from build123d import *

# Parameters (mm, degrees)
F0_W     = 29
F0_H     = 20
F0_W_2   = 10
F0_H_2   = 5.5
F0_W_3   = 2
F0_W_4   = 57.5
F0_H_3   = 44
F1_DEPTH = 4
F2_DEPTH = 47
F3_R     = 11
F3_R_2   = 1.5
F4_DEPTH = 25
F6_DEPTH = 12.5
F8_DEPTH = 50
F9_R     = 2.5
F10_R    = 5


with BuildPart() as f1:
    # F0 (on Top) → F1 (new body)
    with BuildSketch(Plane.XY):
        with Locations((15.5, -34)):
            Rectangle(F0_W, F0_H)
        with Locations((15, -34)):
            Rectangle(F0_W_2, F0_H_2, mode=Mode.SUBTRACT)
        Polygon((1, -24), (30, -24), (30, 24), (1, 24), (-1, 24), (-30, 24), (-30, 22), (27.5, 22), (27.5, -22), (-30, -22), (-30, -24), (-1, -24), align=None)
        with Locations((0, -34)):
            Rectangle(F0_W_3, F0_H)
        with Locations((15.5, 34)):
            Rectangle(F0_W, F0_H)
        with Locations((15, 34)):
            Rectangle(F0_W_2, F0_H_2, mode=Mode.SUBTRACT)
        with Locations((-15.5, -34)):
            Rectangle(F0_W, F0_H)
        with Locations((-15, -34)):
            Rectangle(F0_W_2, F0_H_2, mode=Mode.SUBTRACT)
        with Locations((0, 34)):
            Rectangle(F0_W_3, F0_H)
        with Locations((-15.5, 34)):
            Rectangle(F0_W, F0_H)
        with Locations((-15, 34)):
            Rectangle(F0_W_2, F0_H_2, mode=Mode.SUBTRACT)
        with Locations((-1.25, 0)):
            Rectangle(F0_W_4, F0_H_3)
    extrude(amount=F1_DEPTH)

    # F0 (on Top) → F2 (join)
    with BuildSketch(Plane.XY):
        Polygon((1, -24), (30, -24), (30, 24), (1, 24), (-1, 24), (-30, 24), (-30, 22), (27.5, 22), (27.5, -22), (-30, -22), (-30, -24), (-1, -24), align=None)
        with Locations((0, 34)):
            Rectangle(F0_W_3, F0_H)
        with Locations((0, -34)):
            Rectangle(F0_W_3, F0_H)
    extrude(amount=F2_DEPTH)

    # F3 (on face) → F4 (cut)
    with BuildSketch(Plane.YZ.offset(30)):
        with Locations((0, 25.5)):
            Circle(F3_R)
        with Locations((-15.5, 41)):
            Circle(F3_R_2)
        with Locations((15.5, 41)):
            Circle(F3_R_2)
        with Locations((15.5, 10)):
            Circle(F3_R_2)
        with Locations((-15.5, 10)):
            Circle(F3_R_2)
    extrude(amount=-F4_DEPTH, mode=Mode.SUBTRACT)

    # F5 (on Right) → F6 (cut, symmetric)
    with BuildSketch(Plane.YZ):
        Polygon((-44, 47), (-44, 4), (-34, 25.5), (-24, 47), align=None)
        Polygon((-24, 47), (-34, 25.5), (-24, 25.5), align=None)
        Polygon((34, 25.5), (44, 4), (44, 47), (24, 47), align=None)
        Polygon((24, 25.5), (34, 25.5), (24, 47), align=None)
    extrude(amount=F6_DEPTH, both=True, mode=Mode.SUBTRACT)

    # F7 (on Front) → F8 (cut, symmetric)
    with BuildSketch(Plane.XZ):
        Polygon((-30, 47), (-30, 4), (22.5, 47), align=None)
    extrude(amount=F8_DEPTH, both=True, mode=Mode.SUBTRACT)

    # F9
    f9_edges = [f1.edges().sort_by_distance(p)[0] for p in [
        (-20, 36.75, 2),
        (-20, 31.25, 2),
        (-10, 36.75, 2),
        (-10, 31.25, 2),
        (20, 31.25, 2),
        (20, -36.75, 2),
        (-10, -36.75, 2),
        (20, -31.25, 2),
        (-10, -31.25, 2),
        (20, 36.75, 2),
        (-20, -36.75, 2),
        (10, -36.75, 2),
        (10, 31.25, 2),
        (-20, -31.25, 2),
        (10, -31.25, 2),
        (10, 36.75, 2),
    ]]
    fillet(f9_edges, radius=F9_R)

    # F10
    f10_edges = [f1.edges().sort_by_distance(p)[0] for p in [
        (-30, -44, 2),
        (30, -44, 2),
        (30, 44, 2),
        (-30, 44, 2),
    ]]
    fillet(f10_edges, radius=F10_R)


solid = f1.part
The listing builds one solid part. Answer for the finished solid, in the listing's coordinates (mm). A direction names the side the tool comes from. Coordinates: 2 decimals unless noted, no trailing zeros. Loops run counter-clockwise (first coordinate to the right, second up) from the corner with the lowest first, then second, coordinate; pieces in that order, holes last. Notation, with made-up numbers: M 43.5,39.5 L 81.5,39.5 A13 cw 81.5,49.5 Z; hole C 66.5,-19 d3. An arc over 180 degrees is marked long. Answer in a Markdown table with one row per item.
1) Find the intervals of material crossed by probe 1 along Y at (x, z) = (-16, 3); probe 2 along Z at (x, y) = (28, -15.5); probe 3 along Y at (x, z) = (27, 9), in increasing order.
Answers below:
| item | result |
|---|---|
| probe 1 | -44 to -36.75, -31.25 to 31.25, 36.75 to 44 |
| probe 2 | 0 to 8.5, 11.5 to 39.5, 42.5 to 47 |
| probe 3 | -24 to -22, 22 to 24 |
2) Find section A-A (y = 15.5). Determine the outline of the cut face in (x, z).
Answers below:
| item | result |
|---|---|
| outline | M -30,0 L 30,0 L 30,8.5 L 27.5,8.5 L 27.5,4 L -30,4 Z; M 27.5,11.5 L 30,11.5 L 30,39.5 L 27.5,39.5 Z; M 27.5,42.5 L 30,42.5 L 30,47 L 27.5,47 Z |
3) Find section B-B (y = 0). Determine the outline of the cut face in (x, z).
Answers below:
| item | result |
|---|---|
| outline | M -30,0 L 30,0 L 30,14.5 L 27.5,14.5 L 27.5,4 L -30,4 Z; M 27.5,36.5 L 30,36.5 L 30,47 L 27.5,47 Z |
4) Find section C-C (z = 35.5). Determine the outline of the cut face in (x, y), then the cut area to 3 significant figures.
Answers below:
| item | result |
|---|---|
| outline | M 8.46,-24 L 30,-24 L 30,-4.58 L 27.5,-4.58 L 27.5,-22 L 8.46,-22 Z; M 8.46,22 L 27.5,22 L 27.5,4.58 L 30,4.58 L 30,24 L 8.46,24 Z |
| area | 173 mm^2 |
5) Find section D-D (z = 10). Determine the outline of the cut face in (x, y), then the cut area to 3 significant figures.
Answers below:
| item | result |
|---|---|
| outline | M -22.67,-24 L -1,-24 L -1,-41.21 L 1,-41.21 L 1,-24 L 30,-24 L 30,-17 L 27.5,-17 L 27.5,-22 L -22.67,-22 Z; M -22.67,22 L 27.5,22 L 27.5,17 L 30,17 L 30,24 L 1,24 L 1,41.21 L -1,41.21 L -1,24 L -22.67,24 Z; M 27.5,-14 L 30,-14 L 30,14 L 27.5,14 Z |
| area | 375 mm^2 |
6) Given pin 1 (5 mm diameter, centred on y = 15.5, z = 41, fed in from -X); pin 2 (10 mm diameter, centred on x = -15, y = 34, fed in from +Z); pin 3 (1 mm diameter, centred on x = 23.5, z = 27, fed in from +Y); pin 4 (1.5 mm diameter, centred on y = -32.5, z = 28, fed in from -X), each flat-ended and moving along its own axis, determine where each tip first touches the part or whether it passes through.
Answers below:
| item | result |
|---|---|
| pin 1 | x = 27.5 |
| pin 2 | z = 4 |
| pin 3 | y = 24 |
| pin 4 | through |
7) Which of the six approach directions +Z, -Z, +X, -X, +Y, -Y give full straight-line access (tool end or side, diameter ignored) to faces 1 (the flat face through (-16, -29, 4)), 2 (the flat face through (-4.118, 22.986, 25.199)), 3 (the cylindrical face through (-19.248, -36.037, 2.028)), 4 (the flat face through (5, 22, 20)), 5 (the flat face through (15, 30, 4))?
Answers below:
| item | result |
|---|---|
| face 1 | +Z, -X, -Y |
| face 2 | +Z, -X, +Y, -Y |
| face 3 | +Z, -Z |
| face 4 | +Z, -X |
| face 5 | +Z, +X, +Y |
8) Determine the mould class of faces 6 (the cylindrical face through (-28, 43, 2)), 7 (the cylindrical face through (29, 14, 10)), 8 (the cylindrical face through (19.248, -31.963, 2.028)) for opening direction X: released by +X, released by -X, zero draft, split by the parting line, or undercut.
Answers below:
| item | result |
|---|---|
| face 6 | released by -X |
| face 7 | zero draft |
| face 8 | undercut |
